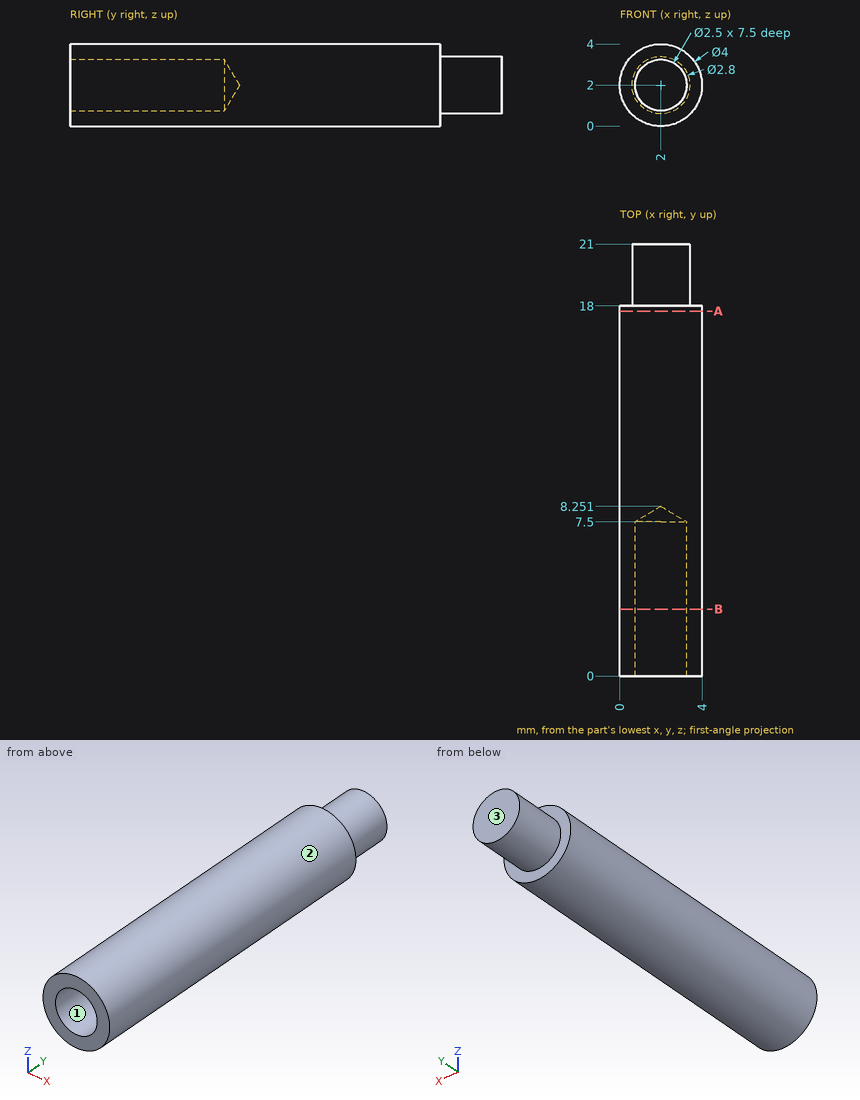
Geometry check sheet. Reference: drawing and pictorial views, mm from the part's lowest x, y, z. Round coordinates to 2 decimals unless told otherwise and drop trailing zeros. Order: outer loops, then holes, each group sorted by start corner. A loop starts at its lowest first (then second) coordinate and runs counter-clockwise, first axis right, second up. Notation, with made-up numbers: M 3.25,37 L 50.25,37 A25 ccw 50.25,67 Z; hole C 8,81.5 d6. An arc over 180 degrees is marked long. Write item = value, one per line.
Q1. Release check for a two-part mould opening along X. For the marked faces 1, 2 and 3 record: released by +X, released by -X, zero draft, split by the parting line, or undercut.
Answer block:
face_1 = undercut
face_2 = split by the parting line
face_3 = zero draft
Q2. Scan lines: line 1 (X direction, y = 5.25, z = 2); line 2 (Y direction, x = 1.6, z = 3.6); line 3 (Z direction, x = 2.5, y = 7.25). Record each from-to range of solid material in increasing order.
Answer block:
line_1 = 0 to 0.75, 3.25 to 4
line_2 = 0 to 18
line_3 = 0.06 to 0.85, 3.15 to 3.94
Q3. Section check B-B (y = 3.25). Enter the section's corners in (x, z).
Answer block:
outline = C 2,2 d4; hole C 2,2 d2.5
Q4. Depth check by flat-ended pin: pin 1 Ø1 at (x, y) = (0.5, 11) entering from -Z; pin 2 Ø2 at (y, z) = (16.5, 3.5) entering from +X. Enter the tip coordinate at first touch or a pass-through.
Answer block:
pin_1 = 0.27
pin_2 = 3.94
Q5. Section check A-A (y = 17.75). Enter the section's corners in (x, z).
Answer block:
outline = C 2,2 d4
